from build123d import *

# Parameters (mm, degrees)
F0_R     = 2.01
F1_DEPTH = 6.35


# Not quite as in the source:
# - a feature names something its author has since deleted; it is built from what else it names


with BuildPart() as f1:
    # F0 (on Front) → F1 (new body)
    with BuildSketch(Plane.XZ):
        Polygon((158, -229.1715728753), (168.5857864376, -218.5857864376), (179.1715728753, -208), (207.5215728753, -208), (207.5215728753, 208), (179.1715728753, 208), (168.5857864376, 218.5857864376), (158, 229.1715728753), (158, 240), (158, 250), (-158, 250), (-158, 240), (-158, 229.1715728753), (-168.5857864376, 218.5857864376), (-179.1715728753, 208), (-207.5215728753, 208), (-207.5215728753, -208), (-179.1715728753, -208), (-168.5857864376, -218.5857864376), (-158, -229.1715728753), (-158, -240), (-158, -250), (158, -250), (158, -240), align=None)
        with Locations((-190, -188)):
            Circle(F0_R, mode=Mode.SUBTRACT)
        with Locations((-138, -240)):
            Circle(F0_R, mode=Mode.SUBTRACT)
        with Locations((0, -240)):
            Circle(F0_R, mode=Mode.SUBTRACT)
        with Locations((138, -240)):
            Circle(F0_R, mode=Mode.SUBTRACT)
        with Locations((190, -188)):
            Circle(F0_R, mode=Mode.SUBTRACT)
        with Locations((-190, 0)):
            Circle(F0_R, mode=Mode.SUBTRACT)
        with Locations((-190, 188)):
            Circle(F0_R, mode=Mode.SUBTRACT)
        with Locations((-138, 240)):
            Circle(F0_R, mode=Mode.SUBTRACT)
        Polygon((-140, 185), (140, 185), (160, 165), (160, -115), (0, -115), (-160, -115), (-160, 165), align=None, mode=Mode.SUBTRACT)
        with Locations((190, 0)):
            Circle(F0_R, mode=Mode.SUBTRACT)
        with Locations((0, 240)):
            Circle(F0_R, mode=Mode.SUBTRACT)
        with Locations((138, 240)):
            Circle(F0_R, mode=Mode.SUBTRACT)
        with Locations((190, 188)):
            Circle(F0_R, mode=Mode.SUBTRACT)
    extrude(amount=F1_DEPTH)


solid = f1.part
The listing builds one solid part. Answer for the finished solid, in the listing's coordinates (mm). A direction names the side the tool comes from. Give positions to 0.01 mm unless a question says otherwise; leave off trailing zeros. Loops run counter-clockwise (first coordinate to the right, second up) from the corner with the lowest first, then second, coordinate; pieces in that order, holes last. Notation, with made-up numbers: (75.5, 49.5) - (121.5, 49.5) arc R10 cw to (121.5, 61.5) - close; hole circle Ø4 at (54.5, 28.5). An arc over 180 degrees is marked (long way). Use one line per item in the form item = value.
1. Section A-A on x = 115 is taken. Give the vertices of the cut face in (y, z), then the cut area to 3 significant figures.
Calculated:
outline = (-6.35, -250) - (0, -250) - (0, -115) - (-6.35, -115) - close; (-6.35, 185) - (0, 185) - (0, 250) - (-6.35, 250) - close
area = 1,270 mm^2
2. Given pin 1 Ø2.5 at (x, z) = (190, 188) entering from +Y; pin 2 Ø1.9 at (y, z) = (-4.5, 242.5) entering from +X, each flat-ended and moving along its own axis, determine where each tip first touches the part or whether it passes through.
Calculated:
pin_1 = through
pin_2 = 158
3. Section C-C on y = -5.25 is taken. Count the separate pieces of the cut face and the enclosed holes in it, then the cut area to 3 significant figures.
Calculated:
separate_pieces = 1
enclosed_holes = 13
area = 104,000 mm^2
4. Section B-B on z = -10.5 is taken. Give the vertices of the cut face in (x, y).
Calculated:
outline = (-207.52, -6.35) - (-160, -6.35) - (-160, 0) - (-207.52, 0) - close; (160, -6.35) - (207.52, -6.35) - (207.52, 0) - (160, 0) - close
5. The mould has two halves that part along X. Classify faces 1 (the face through (150, -3, 175)), 2 (the face through (-3, 0, -163)): pulls with the +X half, pulls with the -X half, needs draft (parallel to the pull), parting line crosses it, or undercut.
Calculated:
face_1 = undercut
face_2 = needs draft
6. Find the intervals of material crossed by line 1 along Z through (x, y) = (-138, -2.5); line 2 along X through (y, z) = (-3, 188); line 3 along X through (y, z) = (-1.5, -240), in increasing order. Write a range as [from, to].
Calculated:
line_1 = [-250, -242.01], [-237.99, -115], [185, 237.99], [242.01, 250]
line_2 = [-207.52, -192.01], [-187.99, 187.99], [192.01, 207.52]
line_3 = [-158, -140.01], [-135.99, -2.01], [2.01, 135.99], [140.01, 158]
7. Which of the six approach directions +Z, -Z, +X, -X, +Y, -Y give full straight-line access (tool end or side, diameter ignored) to faces 3 (the face through (-150, -3, 175)), 4 (the face through (-3, -6.35, -163))?
Calculated:
face_3 = +Y, -Y
face_4 = +Z, -Z, +X, -X, -Y
